Source: CAD feature listing. Evaluate the final solid. Frame: model axes, mm. A direction names the side the tool comes from. Round coordinates to 2 decimals unless told otherwise and drop trailing zeros. Order: outer loops, then holes, each group sorted by start corner. A loop starts at its lowest first (then second) coordinate and runs counter-clockwise, first axis right, second up. Notation, with made-up numbers: M -22,-38 L 24,-38 A35 ccw 24,-1 Z; hole C 56,88.5 d3. An arc over 180 degrees is marked long. Answer in a Markdown table with one row per item. Add a question column.
```python
from build123d import *

# Parameters (mm, degrees)
SKETCH_1_W          = 86
SKETCH_1_H          = 44.4
EXTRUDE_1_DEPTH     = 19.6
EXTRUDE_2_DEPTH     = 5
SKETCH_3_W          = 83.2
SKETCH_3_H          = 13.4
SKETCH_3_H_2        = 12.8
CUT_EXTRUDE_1_DEPTH = 18.4
FILLET_1_R          = 3
EXTRUDE_3_DEPTH     = 0.2


with BuildPart() as part:
    # Эскиз1 → Бобышка-Вытянуть1 (new body)
    with BuildSketch(Plane.XY):
        Rectangle(SKETCH_1_W, SKETCH_1_H)
    extrude(amount=EXTRUDE_1_DEPTH)

    # Эскиз2 → Бобышка-Вытянуть2 (add)
    with BuildSketch(Plane.XY):
        with BuildLine():
            Line((43, 17.2), (43, 13.108775687))
            ThreePointArc((43, 13.108775687), (53.273546839, 0), (43, -13.108775687))
            Line((43, -13.108775687), (43, -17.2))
            ThreePointArc((43, -17.2), (57.273546839, 0), (43, 17.2))
        make_face()
    extrude(amount=EXTRUDE_2_DEPTH)

    # Эскиз3 → Вырез-Вытянуть1 (cut)
    with BuildSketch(Plane.XY.offset(19.6)):
        with Locations((0.2, 14.3)):
            Rectangle(SKETCH_3_W, SKETCH_3_H)
        with Locations((0.2, 0)):
            Rectangle(SKETCH_3_W, SKETCH_3_H_2)
        with Locations((0.2, -14.3)):
            Rectangle(SKETCH_3_W, SKETCH_3_H)
    extrude(amount=-CUT_EXTRUDE_1_DEPTH, mode=Mode.SUBTRACT)

    # Скругление1
    fillet_1_edges = [part.edges().sort_by_distance(p)[0] for p in [
        (-41.4, 21, 10.4),
        (-41.4, -21, 10.4),
        (-43, -22.2, 9.8),
        (-43, 22.2, 9.8),
    ]]
    fillet(fillet_1_edges, radius=FILLET_1_R)

    # Эскиз4 → Бобышка-Вытянуть3 (add)
    with BuildSketch(Plane(origin=(0, 0, 0), x_dir=(-1, 0, 0), z_dir=(0, 0, -1))):
        with BuildLine():
            Line((-50.908934574, 13.500116296), (-28.350220542, 22.2))
            ThreePointArc((-28.350220542, 22.2), (-44.835714922, 31.349521818), (-50.908934574, 13.500116296))
        make_face()
        with BuildLine():
            Line((43, 9.417902962), (28.395750511, 22.2))
            ThreePointArc((28.395750511, 22.2), (46.588074999, 28.251604167), (43, 9.417902962))
        make_face()
        with BuildLine():
            Line((43, -9.417902962), (28.395750511, -22.2))
            ThreePointArc((28.395750511, -22.2), (46.588074999, -28.251604167), (43, -9.417902962))
        make_face()
        with BuildLine():
            Line((-50.908934574, -13.500116296), (-28.350220542, -22.2))
            ThreePointArc((-28.350220542, -22.2), (-44.835714922, -31.349521818), (-50.908934574, -13.500116296))
        make_face()
    extrude(amount=-EXTRUDE_3_DEPTH)


solid = part.part
```
(1) Cut plane C-C (x = 4). Return loops of the section in (y, z).
(2) Line query: line 1 (Y direction, x = 28.5, z = 17.5); line 2 (X direction, y = 14.5, z = 6.25); line 3 (X direction, y = -6.5, z = 9.25). Output: solid intervals per line, ascending. Write a range as from..to.
(3) Cut plane D-D (y = 15). Return loops of the section in (x, z), and give its area (3 significant figures).
(4) Pin query (flat end, axial travel): pin 1 (6 mm diameter, centred on x = 19, z = 14, fed in from +Y); pin 2 (1 mm diameter, centred on x = -29, y = 4.5, fed in from +Z); pin 3 (4.5 mm diameter, centred on x = 51.5, y = -6.5, fed in from +Z). Return the tip coordinate at first contact, or that it passes through.
(5) Draft query along Y for faces 1 (the face through (0, 14, 1.2)), 2 (the face through (3, 0, 0)), 3 (the face through (1, 22.2, 10)). Return one class per face: +Y half, -Y half, draft (parallel to the pull), parting line (faces both ways), or undercut.
(6) Cut plane A-A (y = 4.5). Return loops of the section in (x, z), and give its area (3 significant figures).
(7) Access query for faces 4 (the face through (-41.4, -13, 11)), 5 (the face through (-10, 7, 19.6)), 6 (the face through (-42, -22, 0.2)), 7 (the face through (53.3, -2.5, 5)). Directions: +Z, -Z, +X, -X, +Y, -Y. A direction counts if a zero-diameter tool reaches every point of the face in a straight line with its end or side. Return the directions, or none.
(8) Cut plane B-B (z = 9.5). Return loops of the section in (x, y), and give its area (3 significant figures).
Answer list:
| question | item | result |
|---|---|---|
| 1 | outline | M -22.2,0 L 22.2,0 L 22.2,19.6 L 21,19.6 L 21,1.2 L 7.6,1.2 L 7.6,19.6 L 6.4,19.6 L 6.4,1.2 L -6.4,1.2 L -6.4,19.6 L -7.6,19.6 L -7.6,1.2 L -21,1.2 L -21,19.6 L -22.2,19.6 Z |
| 2 | line 1 | -22.2..-21, -7.6..-6.4, 6.4..7.6, 21..22.2 |
| 2 | line 2 | -43..-41.4, 41.8..43 |
| 2 | line 3 | -43..43 |
| 3 | outline | M -49.25,0 L 51.69,0 L 51.69,0.2 L 48.79,0.2 L 48.79,5 L 43,5 L 43,19.6 L 41.8,19.6 L 41.8,1.2 L -41.4,1.2 L -41.4,19.6 L -43,19.6 L -43,0.2 L -49.25,0.2 Z |
| 3 | area | 185 mm² |
| 4 | pin 1 | y = 22.2 |
| 4 | pin 2 | z = 1.2 |
| 4 | pin 3 | z = 5 |
| 5 | face 1 | undercut |
| 5 | face 2 | draft |
| 5 | face 3 | +Y half |
| 6 | outline | M -43,0 L 43,0 L 43,19.6 L 41.8,19.6 L 41.8,1.2 L -41.4,1.2 L -41.4,19.6 L -43,19.6 Z; M 52.5,0 L 56.69,0 L 56.69,5 L 52.5,5 Z |
| 6 | area | 176 mm² |
| 7 | face 4 | +Z |
| 7 | face 5 | +Z, +X, -X, +Y, -Y |
| 7 | face 6 | +Z, -X, -Y |
| 7 | face 7 | +Z, +X, +Y, -Y |
| 8 | outline | M -43,-19.2 A3 ccw -40,-22.2 L 43,-22.2 L 43,22.2 L -40,22.2 A3 ccw -43,19.2 Z; hole M -41.4,-18 A3 ccw -38.4,-21 L 41.8,-21 L 41.8,-7.6 L -41.4,-7.6 Z; hole M -41.4,-6.4 L 41.8,-6.4 L 41.8,6.4 L -41.4,6.4 Z; hole M -41.4,7.6 L 41.8,7.6 L 41.8,21 L -38.4,21 A3 ccw -41.4,18 Z |
| 8 | area | 524 mm² |
